from build123d import *

# Parameters (mm, degrees)
SKETCH1_W           = 75
SKETCH1_H           = 90
SKETCH1_W_2         = 50
SKETCH1_H_2         = 13
BOSS_EXTRUDE1_DEPTH = 8
FILLET2_R           = 10
FILLET3_R           = 10
FILLET4_R           = 10
SKETCH7_W           = 5
SKETCH7_H           = 34
BOSS_EXTRUDE3_DEPTH = 63
FILLET5_R           = 5
FILLET6_R           = 5
FILLET7_R           = 5
SKETCH2_R           = 16
CUT_EXTRUDE1_DEPTH  = 1
CUT_EXTRUDE2_REACH  = 43
SKETCH8_R           = 2.5
SKETCH8_R_2         = 4


with BuildPart() as part:
    # Sketch1 → Boss-Extrude1 (new body)
    with BuildSketch(Plane(origin=(0, 0, 0), x_dir=(1, 0, 0), z_dir=(0, 1, 0))):
        with Locations((37.5, -45)):
            Rectangle(SKETCH1_W, SKETCH1_H)
        with Locations((100, -83.5)):
            Rectangle(SKETCH1_W_2, SKETCH1_H_2)
    extrude(amount=BOSS_EXTRUDE1_DEPTH)

    # Fillet2
    fillet2_edges = [part.edges().sort_by_distance(p)[0] for p in [
        (0, 4, 0),
    ]]
    fillet(fillet2_edges, radius=FILLET2_R)

    # Fillet3
    fillet3_edges = [part.edges().sort_by_distance(p)[0] for p in [
        (0, 4, 90),
    ]]
    fillet(fillet3_edges, radius=FILLET3_R)

    # Fillet4
    fillet4_edges = [part.edges().sort_by_distance(p)[0] for p in [
        (75, 4, 0),
    ]]
    fillet(fillet4_edges, radius=FILLET4_R)

    # Sketch7 → Boss-Extrude3 (add)
    with BuildSketch(Plane(origin=(125, 0, 0), x_dir=(0, 0, -1), z_dir=(1, 0, 0))):
        with Locations((-87.5, 25)):
            Rectangle(SKETCH7_W, SKETCH7_H)
    extrude(amount=-BOSS_EXTRUDE3_DEPTH)

    # Fillet5
    fillet5_edges = [part.edges().sort_by_distance(p)[0] for p in [
        (125, 42, 87.5),
    ]]
    fillet(fillet5_edges, radius=FILLET5_R)

    # Fillet6
    fillet6_edges = [part.edges().sort_by_distance(p)[0] for p in [
        (125, 4, 77),
    ]]
    fillet(fillet6_edges, radius=FILLET6_R)

    # Fillet7
    fillet7_edges = [part.edges().sort_by_distance(p)[0] for p in [
        (62, 42, 87.5),
    ]]
    fillet(fillet7_edges, radius=FILLET7_R)

    # Sketch2 → Cut-Extrude1 (cut)
    with BuildSketch(Plane.XZ):
        with Locations((37.5, 45)):
            Circle(SKETCH2_R)
    extrude(amount=-CUT_EXTRUDE1_DEPTH, mode=Mode.SUBTRACT)

    # Sketch8 → Cut-Extrude2 (cut, up to next)
    with BuildSketch(Plane.XZ.offset(-1), mode=Mode.PRIVATE) as cut_extrude2_sk1:
        with Locations((37.5, 57)):
            Circle(SKETCH8_R)
    cut_extrude2_tool1 = extrude(cut_extrude2_sk1.sketch, amount=-CUT_EXTRUDE2_REACH, mode=Mode.PRIVATE) & part.part
    add(cut_extrude2_tool1.solids().sort_by_distance((37.5, 1, 57))[0], mode=Mode.SUBTRACT)
    # Sketch8 → Cut-Extrude2 (cut, up to next)
    with BuildSketch(Plane.XZ.offset(-1), mode=Mode.PRIVATE) as cut_extrude2_sk2:
        with Locations((37.5, 45)):
            Circle(SKETCH8_R_2)
    cut_extrude2_tool2 = extrude(cut_extrude2_sk2.sketch, amount=-CUT_EXTRUDE2_REACH, mode=Mode.PRIVATE) & part.part
    add(cut_extrude2_tool2.solids().sort_by_distance((37.5, 1, 45))[0], mode=Mode.SUBTRACT)
    # Sketch8 → Cut-Extrude2 (cut, up to next)
    with BuildSketch(Plane.XZ.offset(-1), mode=Mode.PRIVATE) as cut_extrude2_sk3:
        with Locations((49.5, 45)):
            Circle(SKETCH8_R)
    cut_extrude2_tool3 = extrude(cut_extrude2_sk3.sketch, amount=-CUT_EXTRUDE2_REACH, mode=Mode.PRIVATE) & part.part
    add(cut_extrude2_tool3.solids().sort_by_distance((49.5, 1, 45))[0], mode=Mode.SUBTRACT)
    # Sketch8 → Cut-Extrude2 (cut, up to next)
    with BuildSketch(Plane.XZ.offset(-1), mode=Mode.PRIVATE) as cut_extrude2_sk4:
        with Locations((37.5, 33)):
            Circle(SKETCH8_R)
    cut_extrude2_tool4 = extrude(cut_extrude2_sk4.sketch, amount=-CUT_EXTRUDE2_REACH, mode=Mode.PRIVATE) & part.part
    add(cut_extrude2_tool4.solids().sort_by_distance((37.5, 1, 33))[0], mode=Mode.SUBTRACT)
    # Sketch8 → Cut-Extrude2 (cut, up to next)
    with BuildSketch(Plane.XZ.offset(-1), mode=Mode.PRIVATE) as cut_extrude2_sk5:
        with Locations((25.5, 45)):
            Circle(SKETCH8_R)
    cut_extrude2_tool5 = extrude(cut_extrude2_sk5.sketch, amount=-CUT_EXTRUDE2_REACH, mode=Mode.PRIVATE) & part.part
    add(cut_extrude2_tool5.solids().sort_by_distance((25.5, 1, 45))[0], mode=Mode.SUBTRACT)


solid = part.part
Build history of the part. All positions in model axes, mm. A direction names the side the tool comes from. Give positions to 0.01 mm unless a question says otherwise; leave off trailing zeros. Order: outer loops, then holes, each group sorted by start corner. A loop starts at its lowest first (then second) coordinate and runs counter-clockwise, first axis right, second up. Notation, with made-up numbers: M -11,43.25 L 37,43.25 A34 ccw 37,76.25 Z; hole C 12,-15.5 d10. An arc over 180 degrees is marked long. Use one line per item in the form item = value.
1) Saw through at D-D (z = 33). Give the cut face in (x, y), plus the area to 3 significant figures.
Calculated:
outline = M 0,0 L 26.92,0 L 26.92,1 L 35,1 L 35,8 L 0,8 Z; M 40,1 L 48.08,1 L 48.08,0 L 75,0 L 75,8 L 40,8 Z
area = 544 mm2
2) Tool access for faces 4 (the face through (75, 4, 44)), 5 (the face through (62, 23, 88)), 6 (the face through (41, 1, 42)), 7 (the face through (94, 25, 85)): list every direction of +Z, -Z, +X, -X, +Y, -Y with a clear straight run to the whole face (end or side of a thin tool).
Calculated:
face_4 = -Z, +X, +Y, -Y
face_5 = +Z, -Z, -X, +Y
face_6 = -Y
face_7 = -Z, +X, -X, +Y
3) Saw through at C-C (y = 6). Give the cut face in (x, z).
Calculated:
outline = M 0,10 A10 ccw 10,0 L 65,0 A10 ccw 75,10 L 75,77 L 120,77 A5 ccw 125,82 L 125,90 L 10,90 A10 ccw 0,80 Z; hole C 25.5,45 d5; hole C 37.5,45 d8; hole C 37.5,33 d5; hole C 37.5,57 d5; hole C 49.5,45 d5
4) Drop flat-ended pins along their axis: pin 1 (6 mm diameter, centred on x = 25.5, z = 45, fed in from -Y); pin 2 (4.5 mm diameter, centred on x = 37.5, z = 57, fed in from +Y); pin 3 (2.5 mm diameter, centred on x = 91.5, y = 4, fed in from -Z); pin 4 (6 mm diameter, centred on x = 49.5, z = 45, fed in from +Y). Give the stop position or say it passes through.
Calculated:
pin_1 = 1
pin_2 = through
pin_3 = 77
pin_4 = 8
5) Probe probe 1 along Z at (x, y) = (37.5, 5); probe 2 along Y at (x, z) = (17, 37.5); probe 3 along Z at (x, y) = (37.5, 0.2). List the from-to ranges inside material, lowest first.
Calculated:
probe_1 = 0 to 30.5, 35.5 to 41, 49 to 54.5, 59.5 to 90
probe_2 = 0 to 8
probe_3 = 0 to 29, 61 to 90
6) Two-plate mould, pull along X, no slides. Class faces 1 (the face through (124, 4, 79)), 2 (the face through (21.515, 0.493, 45.703)), 3 (the face through (2.85, 4.06, 86.99)): released by +X, released by -X, zero draft, split by the parting line, or undercut.
Calculated:
face_1 = released by +X
face_2 = undercut
face_3 = released by -X
7) Saw through at B-B (x = 37.5). Give the cut face in (y, z).
Calculated:
outline = M 0,0 L 8,0 L 8,30.5 L 1,30.5 L 1,29 L 0,29 Z; M 0,61 L 1,61 L 1,59.5 L 8,59.5 L 8,90 L 0,90 Z; M 1,35.5 L 8,35.5 L 8,41 L 1,41 Z; M 1,49 L 8,49 L 8,54.5 L 1,54.5 Z
8) Saw through at A-A (z = 45). Give the cut face in (x, y), plus the area to 3 significant figures.
Calculated:
outline = M 0,0 L 21.5,0 L 21.5,1 L 23,1 L 23,8 L 0,8 Z; M 28,1 L 33.5,1 L 33.5,8 L 28,8 Z; M 41.5,1 L 47,1 L 47,8 L 41.5,8 Z; M 52,1 L 53.5,1 L 53.5,0 L 75,0 L 75,8 L 52,8 Z
area = 442 mm2
